```python
from build123d import *

# Parameters (mm, degrees)
F0_R     = 6
F1_DEPTH = 2.5
F2_DEPTH = 8
F3_R     = 1.54


with BuildPart() as f1:
    # F0 (on Front) → F1 (new body)
    with BuildSketch(Plane.XZ):
        with BuildLine():
            ThreePointArc((-20, -9.96), (-19.256051, -11.756051), (-17.46, -12.5))
            Line((-17.46, -12.5), (17.46, -12.5))
            ThreePointArc((17.46, -12.5), (19.256051, -11.756051), (20, -9.96))
            Line((20, -9.96), (20, 8.970588))
            ThreePointArc((20, 8.970588), (19.695671, 12.446295), (18.791946, 15.816226))
            Line((18.791946, 15.816226), (13.154362, 31.291946))
            ThreePointArc((13.154362, 31.291946), (0, 40.5), (-13.154362, 31.291946))
            Line((-13.154362, 31.291946), (-18.791946, 15.816226))
            ThreePointArc((-18.791946, 15.816226), (-19.695671, 12.446295), (-20, 8.970588))
            Line((-20, 8.970588), (-20, -9.96))
        make_face()
        with BuildLine():
            ThreePointArc((-15.5, -7.5), (-17, -6), (-15.5, -4.5))
            Line((-15.5, -4.5), (15.5, -4.5))
            ThreePointArc((15.5, -4.5), (17, -6), (15.5, -7.5))
            Line((15.5, -7.5), (-15.5, -7.5))
        make_face(mode=Mode.SUBTRACT)
        with BuildLine():
            Line((15.5, 4.5), (-15.5, 4.5))
            ThreePointArc((-15.5, 4.5), (-17, 6), (-15.5, 7.5))
            Line((-15.5, 7.5), (15.5, 7.5))
            ThreePointArc((15.5, 7.5), (17, 6), (15.5, 4.5))
        make_face(mode=Mode.SUBTRACT)
        with Locations((0, 26.5)):
            Circle(F0_R, mode=Mode.SUBTRACT)
    extrude(amount=F1_DEPTH)


with BuildPart() as f2:
    # F0 (on Front) → F2 (new body)
    with BuildSketch(Plane.XZ):
        with Locations((0, 26.5)):
            Circle(F0_R)
    extrude(amount=F2_DEPTH)

    # F3
    f3_edges = [f2.edges().sort_by_distance(p)[0] for p in [
        (-6, -8, 26.5),
    ]]
    fillet(f3_edges, radius=F3_R)


solid = f1.part
```
The model under review builds one solid part; all positions refer to its coordinate system, in mm. A direction names the side the tool comes from. Give positions to 0.01 mm unless a question says otherwise; leave off trailing zeros. Write each loop counter-clockwise with the first axis right and the second up, starting at its lowest first coordinate (ties: lowest second). Pieces come first, ordered by that corner, then holes. Notation, with made-up numbers: (0, 76) -> (30, 76) arc R35 cw to (30, 108) -> close; hole circle Ø5 at (74.25, 27.5). An arc over 180 degrees is marked (long way). Answer in a Markdown table with one row per item.
1) Add section A-A on x = 14. State the section outline as (y, z) points, plus the area to 3 significant figures.
Worked answers:
| item | result |
|---|---|
| outline | (-2.5, -12.5) -> (0, -12.5) -> (0, -7.5) -> (-2.5, -7.5) -> close; (-2.5, -4.5) -> (0, -4.5) -> (0, 4.5) -> (-2.5, 4.5) -> close; (-2.5, 7.5) -> (0, 7.5) -> (0, 28.97) -> (-2.5, 28.97) -> close |
| area | 88.7 mm² |
2) Add section D-D on x = -4.5. State the section outline as (y, z) points.
Worked answers:
| item | result |
|---|---|
| outline | (-2.5, -12.5) -> (0, -12.5) -> (0, -7.5) -> (-2.5, -7.5) -> close; (-2.5, -4.5) -> (0, -4.5) -> (0, 4.5) -> (-2.5, 4.5) -> close; (-2.5, 7.5) -> (0, 7.5) -> (0, 22.53) -> (-2.5, 22.53) -> close; (-2.5, 30.47) -> (0, 30.47) -> (0, 39.76) -> (-2.5, 39.76) -> close |
3) For L1, parallel to Z at x = 11, y = -1.8; L2, parallel to Z at x = -5, y = -2.3; L3, parallel to Z at x = -9.5, y = -1.4, list the stretches that pass through material, from the lowest coordinate up. Write a range as [from, to].
Worked answers:
| item | result |
|---|---|
| L1 | [-12.5, -7.5], [-4.5, 4.5], [7.5, 35.16] |
| L2 | [-12.5, -7.5], [-4.5, 4.5], [7.5, 23.18], [29.82, 39.58] |
| L3 | [-12.5, -7.5], [-4.5, 4.5], [7.5, 36.78] |
4) Add section B-B on z = -6. State the section outline as (x, y) points.
Worked answers:
| item | result |
|---|---|
| outline | (-20, -2.5) -> (-17, -2.5) -> (-17, 0) -> (-20, 0) -> close; (17, -2.5) -> (20, -2.5) -> (20, 0) -> (17, 0) -> close |
5) Clearance check with a flat-ended pin moving along its axis: P1, Ø1, axis at y = -2, z = 11, coming from the +X side. State where the tip first meets the part, or that it passes through.
Worked answers:
| item | result |
|---|---|
| P1 | x = 19.94 |
6) Mouldability with a two-part tool opening along Z and no side actions: class faces 1 (the flat face through (20, -1, -1)), 2 (the flat face through (0, -1, -7.5)), 3 (the cylindrical face through (-17, -1, -6)), 4 (the cylindrical face through (-19.276, -1.232, -11.736)) as +Z half, -Z half, draft (parallel to the pull), parting line (faces both ways), or undercut.
Worked answers:
| item | result |
|---|---|
| face 1 | draft |
| face 2 | undercut |
| face 3 | undercut |
| face 4 | -Z half |
7) Add section C-C on y = -2.05. State the section outline as (x, z) points.
Worked answers:
| item | result |
|---|---|
| outline | (-20, -9.96) arc R2.54 ccw to (-17.46, -12.5) -> (17.46, -12.5) arc R2.54 ccw to (20, -9.96) -> (20, 8.97) arc R20 ccw to (18.79, 15.82) -> (13.15, 31.29) arc R14 ccw to (-13.15, 31.29) -> (-18.79, 15.82) arc R20 ccw to (-20, 8.97) -> close; hole (-15.5, -7.5) -> (15.5, -7.5) arc R1.5 ccw to (15.5, -4.5) -> (-15.5, -4.5) arc R1.5 ccw to start; hole (-15.5, 4.5) -> (15.5, 4.5) arc R1.5 ccw to (15.5, 7.5) -> (-15.5, 7.5) arc R1.5 ccw to start; hole circle Ø12 at (0, 26.5) |
8) Tool access review of faces 5 (the cylindrical face through (17, -1, 6)), 6 (the flat face through (-20, -1, 0)): name each direction out of +Z, -Z, +X, -X, +Y, -Y from which nothing blocks a thin tool from reaching the whole face with its end or side.
Worked answers:
| item | result |
|---|---|
| face 5 | +Y, -Y |
| face 6 | +Z, -Z, -X, +Y, -Y |
